Verification items for the finished model (mm, model axes). A direction names the side the tool comes from. Coordinates: 2 decimals unless noted, no trailing zeros. Write each loop counter-clockwise with the first axis right and the second up, starting at its lowest first coordinate (ties: lowest second). Pieces come first, ordered by that corner, then holes. Notation, with made-up numbers: M 86,76.5 L 133,76.5 A28 ccw 133,107.5 Z; hole C 46,-15 d10. An arc over 180 degrees is marked long. Answer in a Markdown table with one row per item.
from build123d import *

# Parameters (mm, degrees)
SKETCH_1_R          = 22.5
SKETCH_1_R_2        = 20.5
EXTRUDE_1_DEPTH     = 5
EXTRUDE_START       = -5
SKETCH_1_4_R        = 22.5
EXTRUDE_2_DEPTH     = 5
SKETCH_2_R          = 5.1
CUT_EXTRUDE_1_DEPTH = 1.5
SKETCH_3_W          = 30
SKETCH_3_H          = 5
CUT_EXTRUDE_2_DEPTH = 5
SKETCH_4_R          = 0.6
CUT_EXTRUDE_3_DEPTH = 3


with BuildPart() as part:
    # 草图1 → 凸台-拉伸1 (new body)
    with BuildSketch(Plane(origin=(0, 0, 0), x_dir=(1, 0, 0), z_dir=(0, 1, 0))):
        with Locations(Location((0, 0, 0), (0, 0, 270))):
            Circle(SKETCH_1_R)
        with Locations(Location((0, 0, 0), (0, 0, 270))):
            Circle(SKETCH_1_R_2, mode=Mode.SUBTRACT)
    extrude(amount=EXTRUDE_1_DEPTH)

    # 草图1<4> → 凸台-拉伸2 (add)
    with BuildSketch(Plane(origin=(0, 0, 0), x_dir=(1, 0, 0), z_dir=(0, 1, 0)).offset(EXTRUDE_START)):
        with Locations(Location((0, 0, 0), (0, 0, 270))):
            Circle(SKETCH_1_4_R)
    extrude(amount=EXTRUDE_2_DEPTH)

    # 草图2 → 切除-拉伸1 (cut)
    with BuildSketch(Plane(origin=(0, 0, 0), x_dir=(1, 0, 0), z_dir=(0, 1, 0))):
        with Locations(Location((0, 9.7, 0), (0, 0, 270))):
            Circle(SKETCH_2_R)
        with Locations((-5, -9.7)):
            Circle(SKETCH_2_R)
        with Locations((5, -9.7)):
            Circle(SKETCH_2_R)
    extrude(amount=-CUT_EXTRUDE_1_DEPTH, mode=Mode.SUBTRACT)

    # 草图3 → 切除-拉伸2 (cut)
    with BuildSketch(Plane(origin=(0, 5, 0), x_dir=(1, 0, 0), z_dir=(0, 1, 0))):
        with Locations((15, 0)):
            Rectangle(SKETCH_3_W, SKETCH_3_H)
    extrude(amount=-CUT_EXTRUDE_2_DEPTH, mode=Mode.SUBTRACT)

    # 草图4 → 切除-拉伸3 (cut)
    with BuildSketch(Plane.XZ.offset(5)):
        with Locations(Location((-10, 0, 0), (0, 0, 270))):
            Circle(SKETCH_4_R)
        with Locations(Location((10, 0, 0), (0, 0, 270))):
            Circle(SKETCH_4_R)
    extrude(amount=-CUT_EXTRUDE_3_DEPTH, mode=Mode.SUBTRACT)


solid = part.part
1) Sectioned sample at C-C (y = 2). Record the cut outline in (x, z).
Response values:
| item | result |
|---|---|
| outline | M 20.35,-2.5 A20.5 cw long 20.35,2.5 L 22.36,2.5 A22.5 ccw long 22.36,-2.5 Z |
2) Sectioned sample at D-D (z = 16.5). Record the cut outline in (x, y), then the cut area to 3 significant figures.
Response values:
| item | result |
|---|---|
| outline | M -15.3,-5 L 15.3,-5 L 15.3,5 L 12.17,5 L 12.17,0 L -12.17,0 L -12.17,5 L -15.3,5 Z |
| area | 184 mm² |
3) Sectioned sample at B-B (x = -8.5). Record the cut outline in (y, z).
Response values:
| item | result |
|---|---|
| outline | M -5,-20.83 L 5,-20.83 L 5,-18.65 L 0,-18.65 L 0,5.99 L -1.5,5.99 L -1.5,13.41 L 0,13.41 L 0,18.65 L 5,18.65 L 5,20.83 L -5,20.83 Z |
4) Tool access check on faces 1 (the face through (0.224, -0.74, -14.795)), 2 (the face through (-4.9, 5, -20.1)), 3 (the face through (10, -2, 0)), 4 (the face through (21, 3, 2.5)). Record the directions out of +Z, -Z, +X, -X, +Y, -Y that give a thin tool (end or side, any length) a straight path to the whole face; none if there is none.
Response values:
| item | result |
|---|---|
| face 1 | +Y |
| face 2 | +Z, -Z, +X, -X, +Y |
| face 3 | -Y |
| face 4 | +X, +Y |
5) Thickness scan on L1, parallel to X at y = -3.45, z = 0; L2, parallel to Z at x = 0, y = 3.9; L3, parallel to Z at x = -2, y = -1.25. Record the ranges inside material, lowest first. Write a range as [from, to].
Response values:
| item | result |
|---|---|
| L1 | x = [-22.5, -10.6], [-9.4, 9.4], [10.6, 22.5] |
| L2 | z = [-22.5, -20.5], [20.5, 22.5] |
| L3 | z = [-22.41, -14.39], [-5.01, 5.58], [13.82, 22.41] |
6) Release check for a two-part mould opening along X. For faces 5 (the face through (0, -1.5, -10)), 6 (the face through (-10, -2, 0)), 7 (the face through (0, -5, 0)), 8 (the face through (-8.618, -0.07, 20.784)) record: +X half, -X half, draft (parallel to the pull), parting line (faces both ways), or undercut.
Response values:
| item | result |
|---|---|
| face 5 | undercut |
| face 6 | undercut |
| face 7 | draft |
| face 8 | parting line |
7) Sectioned sample at A-A (z = -9.7). Record the cut outline in (x, y).
Response values:
| item | result |
|---|---|
| outline | M -20.3,-5 L 20.3,-5 L 20.3,5 L 18.06,5 L 18.06,0 L 5.1,0 L 5.1,-1.5 L -5.1,-1.5 L -5.1,0 L -18.06,0 L -18.06,5 L -20.3,5 Z |
8) Depth check by flat-ended pin: pin 1 (2 mm diameter, centred on x = -3.5, z = -14.5, fed in from +Y); pin 2 (4 mm diameter, centred on x = -14.5, y = -1.5, fed in from -Z); pin 3 (5 mm diameter, centred on x = 0, z = -9.5, fed in from +Y). Enter the tip coordinate at first touch or a pass-through.
Response values:
| item | result |
|---|---|
| pin 1 | stops at y = 0 |
| pin 2 | stops at z = -18.71 |
| pin 3 | stops at y = -1.5 |
